Part model, mm, in its own coordinate system. Coordinates: 2 decimals unless noted, no trailing zeros. Loops run counter-clockwise (first coordinate to the right, second up) from the corner with the lowest first, then second, coordinate; pieces in that order, holes last. Notation, with made-up numbers: (-13, -4.5) - (-1, -4.5) arc R25 cw to (-1, 15.5) - close; hole circle Ø9 at (31.25, 84). An arc over 180 degrees is marked (long way). Answer as CSV lines item,"result".
from build123d import *

# Parameters (mm, degrees)
SKETCH1_W           = 10
SKETCH1_H           = 12
BOSS_EXTRUDE1_DEPTH = 16
SKETCH2_R           = 1.5
CUT_EXTRUDE1_DEPTH  = 16
SKETCH2_3_R         = 2
CUT_EXTRUDE2_DEPTH  = 8


with BuildPart() as part:
    # Sketch1 → Boss-Extrude1 (new body)
    with BuildSketch(Plane(origin=(0, 0, 0), x_dir=(1, 0, 0), z_dir=(0, 1, 0))):
        Rectangle(SKETCH1_W, SKETCH1_H)
    extrude(amount=BOSS_EXTRUDE1_DEPTH)

    # Sketch2 → Cut-Extrude1 (cut)
    with BuildSketch(Plane(origin=(0, 16, 0), x_dir=(1, 0, 0), z_dir=(0, 1, 0))):
        with Locations(Location((0, -3, 0), (0, 0, 270))):
            Circle(SKETCH2_R)
    extrude(amount=-CUT_EXTRUDE1_DEPTH, mode=Mode.SUBTRACT)

    # Sketch2_3 → Cut-Extrude2 (cut)
    with BuildSketch(Plane(origin=(0, 16, 0), x_dir=(1, 0, 0), z_dir=(0, 1, 0))):
        with Locations(Location((0, -3, 0), (0, 0, 270))):
            Circle(SKETCH2_3_R)
    extrude(amount=-CUT_EXTRUDE2_DEPTH, mode=Mode.SUBTRACT)


solid = part.part
Q1. Saw through at D-D (y = 12). Give the cut face in (x, z).
Results:
outline,"(-5, -6) - (5, -6) - (5, 6) - (-5, 6) - close; hole circle Ø4 at (0, 3)"
Q2. Two-plate mould, pull along Z, no slides. Class faces 1 (the face through (-5, 8, 0)), 2 (the face through (-2, 12, 3)), 3 (the face through (0, 8, -6)): released by +Z, released by -Z, zero draft, split by the parting line, or undercut.
Results:
face 1,"zero draft"
face 2,"undercut"
face 3,"released by -Z"
Q3. Saw through at A-A (x = 0). Give the cut face in (y, z).
Results:
outline,"(0, -6) - (16, -6) - (16, 1) - (8, 1) - (8, 1.5) - (0, 1.5) - close; (0, 4.5) - (8, 4.5) - (8, 5) - (16, 5) - (16, 6) - (0, 6) - close"
Q4. Saw through at C-C (y = 2.5). Give the cut face in (x, z).
Results:
outline,"(-5, -6) - (5, -6) - (5, 6) - (-5, 6) - close; hole circle Ø3 at (0, 3)"
Q5. Saw through at B-B (z = 3). Give the cut face in (x, y), then the cut area to 3 significant figures.
Results:
outline,"(-5, 0) - (-1.5, 0) - (-1.5, 8) - (-2, 8) - (-2, 16) - (-5, 16) - close; (1.5, 0) - (5, 0) - (5, 16) - (2, 16) - (2, 8) - (1.5, 8) - close"
area,"104 mm^2"
Q6. Flat gauge pin, fed straight in: pin 1 (4.5 mm diameter, centred on x = 0, z = 2, fed in from +Y). Where does the tip first touch, or does it go through?
Results:
pin 1,"stops at y = 16"
Q7. Wall check: L1, parallel to X at y = 14.25, z = 3; L2, parallel to Y at x = -1.25, z = 4.5; L3, parallel to Z at x = 0.75, y = 15.25. Give the ranges that are in metal, low to high.
Results:
L1,"x = -5 to -2, 2 to 5"
L2,"y = 0 to 8"
L3,"z = -6 to 1.15, 4.85 to 6"
